Autodesk Inventor part; units mm, degrees
ref_plane "YZ Plane" through (0, 0, 0) normal (1, 0, 0) x (0, 1, 0)
ref_plane "XZ Plane" through (0, 0, 0) normal (0, 1, 0) x (-1, 0, 0)
ref_plane "XY Plane" through (0, 0, 0) normal (0, 0, 1) x (1, 0, 0)
sketch "Sketch1" plane through (0, 0, 0) normal (0, 1, 0) x (-1, 0, 0)
  line L0 (40, 10) -> (40, -20)
  line L1 (40, -20) -> (-40, -20)
  line L2 (-40, -20) -> (-40, 10)
  line L3 (-30, 20) -> (30, 20)
  line L4 (40, 20) -> (-40, -20) construction
  line L5 (40, -20) -> (-40, 20) construction
  arc A0 (40, 10) -> (30, 20) centre (30, 10) ccw
  arc A1 (-30, 20) -> (-40, 10) centre (-30, 10) ccw
  circle A2 centre (30, 10) radius 4
  circle A3 centre (-30, 10) radius 4
  point P0 (0, 0)
  dimension "d0" = 40
  dimension "d1" = 80
  dimension "d2" = 20
  dimension "d3" = 20
  dimension "d4" = 8
  dimension "d5" = 8
extrude "Extrusion1" add sketch "Sketch1" along normal blind 10
sketch "Sketch2" plane through (40, 0, -20) normal (0, 0, -1) x (-1, 0, 0)
  line L0 (70, 10) -> (10, 10)
  line L1 (40, 10) -> (60, 10)
  line L2 (40, 10) -> (20, 10)
  line L3 (60, 10) -> (60, 30)
  line L4 (60, 30) -> (20, 30)
  line L5 (20, 30) -> (20, 10)
  point P0 (40, 0)
  dimension "d8" = 20
  dimension "d9" = 20
  dimension "d10" = 20
extrude "Extrusion2" add sketch "Sketch2" against normal blind 35
sketch "Sketch3" plane through (40, 0, 15) normal (0, 0, 1) x (1, 0, 0)
  line L0 (-20, 30) -> (-60, 30)
  circle A0 centre (-40, 30) radius 15
  point P0 (-40, 0)
  dimension "d13" = 30
extrude "Extrusion3" cut sketch "Sketch3" against normal blind 35
sketch "Sketch4" plane through (40, 0, -20) normal (0, 0, -1) x (-1, 0, 0)
  line L0 (20, 10) -> (20, 30)
  line L1 (20, 30) -> (8.1955, 30)
  circle A0 centre (8, 22) radius 4
  line L2 (0, 10) -> (20, 10)
  line L3 (0, 10) -> (20, 10)
  line L4 (20, 10) -> (20, 30)
  line L5 (0, 10) -> (0, 22)
  line L6 (8, 30) -> (8.1955, 30)
  arc A1 (8, 30) -> (0, 22) centre (8, 22) ccw
  point P0 (40, 0)
  dimension "d17" = 8
  dimension "d18" = 16
extrude "Extrusion4" add sketch "Sketch4" against normal blind 10
mirror "Mirror1" about plane through (0, 0, 0) normal (1, 0, 0) of "Extrusion4"
chamfer "Chamfer1" distance 2 angle 45 1 edges at (-20, 30, 2.5)
sketch "Sketch5" plane through (40, 0, 15) normal (0, 0, 1) x (1, 0, 0)
  circle A0 centre (-40, 30) radius 15
  point P0 (-40, 0)
  point P1 (-25, 30)
extrude "Extrusion5" add sketch "Sketch5" against normal up to surface (35 mm away)
sketch "Sketch6" plane through (40, 0, 15) normal (0, 0, 1) x (1, 0, 0)
  arc A0 (-25, 30) -> (-55, 30) centre (-40, 30) ccw
  circle A1 centre (-40, 30) radius 11.7834
  point P0 (-40, 0)
extrude "Extrusion6" cut sketch "Sketch6" against normal through all
thread "Thread1"
hole "Hole1" at (30.6261, 10, -2.8857) direction (0, -1, 0) diameter 3 end through all countersink diameter 7 countersink angle 90
The model under review builds one solid part; all positions refer to its coordinate system, in mm. A direction names the side the tool comes from. Round coordinates to 2 decimals unless told otherwise and drop trailing zeros. Order: outer loops, then holes, each group sorted by start corner. A loop starts at its lowest first (then second) coordinate and runs counter-clockwise, first axis right, second up. Notation, with made-up numbers: M 73.5,5.25 L 125.5,5.25 A30 ccw 125.5,44.25 Z; hole C -20,-35 d5. An arc over 180 degrees is marked long. Use a Markdown table: item, result.
1) Consider section C-C (x = 0). Write out the cut boundary in (y, z), then the cut area to 3 significant figures.
Report:
| item | result |
|---|---|
| outline | M 0,-20 L 18.22,-20 L 18.22,15 L 10,15 L 10,20 L 0,20 Z; M 41.78,-20 L 45,-20 L 45,15 L 41.78,15 Z |
| area | 800 mm^2 |
2) Tool access review of faces 1 (the face through (0, 16, 15)), 2 (the face through (-21, 30, -11)), 3 (the face through (-29, 18, -10)): name each direction out of +Z, -Z, +X, -X, +Y, -Y from which nothing blocks a thin tool from reaching the whole face with its end or side.
Report:
| item | result |
|---|---|
| face 1 | +Z, +X, -X, +Y |
| face 2 | +Z, -Z, -X, +Y |
| face 3 | +Z, -X, +Y |
3) Consider section A-A (z = 7). Write out the cut boundary in (x, y).
Report:
| item | result |
|---|---|
| outline | M -40,0 L -32.65,0 L -32.65,10 L -40,10 Z; M -27.35,0 L 27.35,0 L 27.35,10 L 20,10 L 20,30 L 15,30 A15 ccw -15,30 L -18,30 L -20,28 L -20,10 L -27.35,10 Z; M 32.65,0 L 40,0 L 40,10 L 32.65,10 Z; hole C 0,30 d23.57 |
4) Consider section D-D (z = -16.5). Write out the cut boundary in (x, y), then the cut area to 3 significant figures.
Report:
| item | result |
|---|---|
| outline | M -40,0 L 40,0 L 40,22 A8 ccw 32,30 L 15,30 A15 ccw -15,30 L -32,30 A8 ccw -40,22 Z; hole C -32,22 d8; hole C 0,30 d23.57; hole C 32,22 d8 |
| area | 2,190 mm^2 |
5) Consider section B-B (y = 23). Write out the cut boundary in (x, z), then the cut area to 3 significant figures.
Report:
| item | result |
|---|---|
| outline | M -39.94,-20 L -35.87,-20 L -35.87,-10 L -39.94,-10 Z; M -28.13,-20 L -9.48,-20 L -9.48,15 L -20,15 L -20,-10 L -28.13,-10 Z; M 9.48,-20 L 28.13,-20 L 28.13,-10 L 20,-10 L 20,15 L 9.48,15 Z; M 35.87,-20 L 39.94,-20 L 39.94,-10 L 35.87,-10 Z |
| area | 980 mm^2 |
6) Draft analysis for pull direction X (two halves, no side actions). For faces 4 (the face through (-37.719, 27.594, -15.07)), 5 (the face through (0, 5, 20)), 6 (the face through (20, 20, 2)), 7 (the face through (33.2, 4.9, 12.4)), state which applies: released by +X, released by -X, zero draft, split by the parting line, or undercut.
Report:
| item | result |
|---|---|
| face 4 | released by -X |
| face 5 | zero draft |
| face 6 | released by +X |
| face 7 | undercut |
7) Wall thickness on line 1 along Y through (x, z) = (32, -18); line 2 along Z through (x, y) = (-30, 5); line 3 along Z through (x, y) = (30, 2.25): over which ranges is each line inside the solid? List them lowest first. Write a range as [from, to].
Report:
| item | result |
|---|---|
| line 1 | [0, 18], [26, 30] |
| line 2 | [-20, 6], [14, 20] |
| line 3 | [-20, -4.25], [-1.52, 6], [14, 20] |
8) Insertion check: pin 1 (10 mm diameter, centred on x = 30.5, y = 16.5, fed in from +Z); pin 2 (10 mm diameter, centred on x = 14.5, z = -5, fed in from +Y); pin 3 (17.5 mm diameter, centred on x = -5, y = 24.5, fed in from +Z). Each pin has a flat end and moves straight along its axis. Give the tip position at first contact, or say it passes through.
Report:
| item | result |
|---|---|
| pin 1 | z = -10 |
| pin 2 | y = 41.61 |
| pin 3 | z = 15 |
